Geometry: see drawing. Coordinates: mm, zero at the bounding-box minimum. Coordinates: 2 decimals unless noted, no trailing zeros. Write each loop counter-clockwise with the first axis right and the second up, starting at its lowest first coordinate (ties: lowest second). Pieces come first, ordered by that corner, then holes. Notation, with made-up numbers: (36, -4.75) - (42, -4.75) arc R25 ccw to (42, 32.25) - close; hole circle Ø7 at (-11, 29). An arc over 180 degrees is marked (long way). Use CSV: the item, a comma, the result in double quotes.
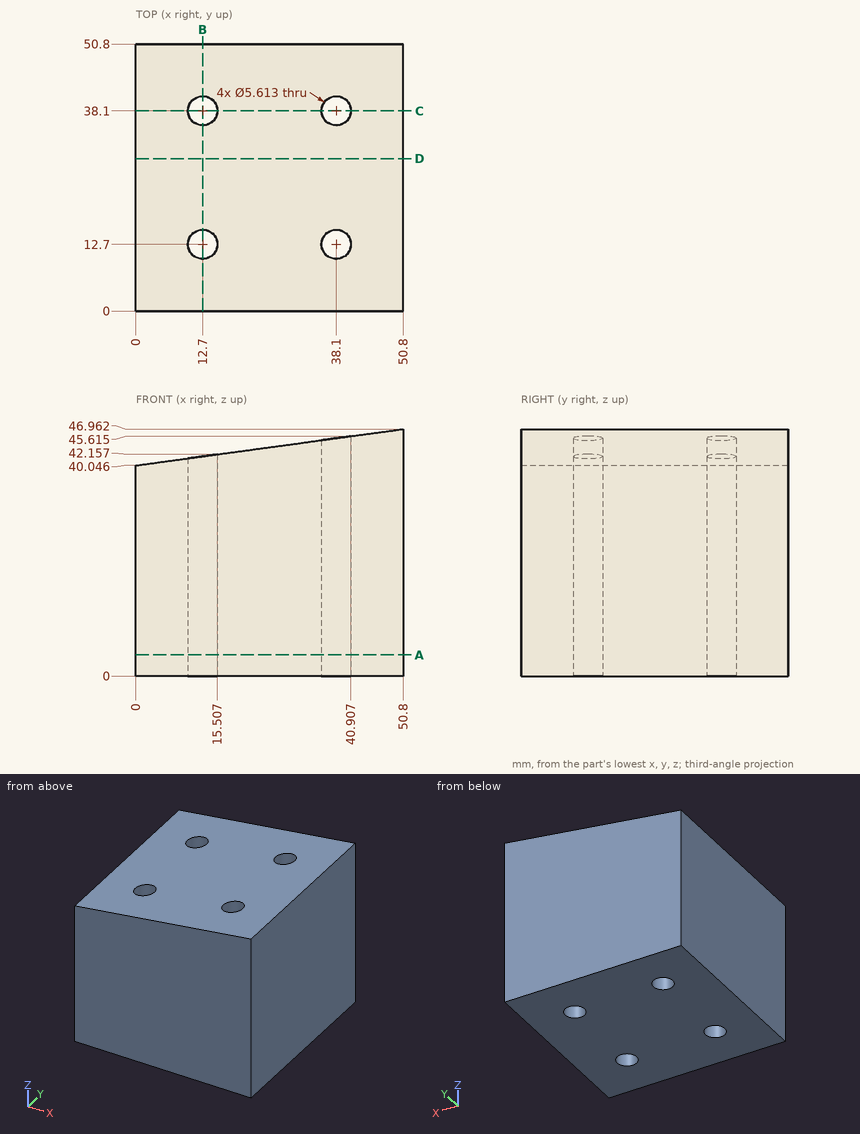
(1) Cut plane C-C on y = 38.1. State how many separate pieces and enclosed holes the cut face has, and give its area (3 significant figures).
Check values:
separate pieces,"3"
enclosed holes,"0"
area,"1,720 mm^2"
(2) Ray query, probe 1 along X at (y, z) = (12.7, 26); probe 2 along Y at (x, z) = (14, 38). Return the intervals inside material, ascending. Write a range as from..to.
Check values:
probe 1,"0..9.89, 15.51..35.29, 40.91..50.8"
probe 2,"0..10.21, 15.19..35.61, 40.59..50.8"
(3) Cut plane D-D on y = 29. Return loops of the section in (x, z), and give its area (3 significant figures).
Check values:
outline,"(0, 0) - (50.8, 0) - (50.8, 46.96) - (0, 40.05) - close"
area,"2,210 mm^2"
(4) Cut plane A-A on z = 4. Return loops of the section in (x, y), and give its area (3 significant figures).
Check values:
outline,"(0, 0) - (50.8, 0) - (50.8, 50.8) - (0, 50.8) - close; hole circle Ø5.61 at (12.7, 12.7); hole circle Ø5.61 at (12.7, 38.1); hole circle Ø5.61 at (38.1, 12.7); hole circle Ø5.61 at (38.1, 38.1)"
area,"2,480 mm^2"
(5) Pin query (flat end, axial travel): pin 1 Ø6.5 at (x, y) = (12.7, 38.1) entering from +Z; pin 2 Ø5 at (x, y) = (10, 36) entering from +Z (1 decimal); pin 3 Ø5 at (x, y) = (28.5, 16.5) entering from +Z. Return the tip coordinate at first contact, or that it passes through.
Check values:
pin 1,"z = 42.22"
pin 2,"z = 41.7"
pin 3,"z = 44.27"
(6) Cut plane B-B on x = 12.7. Return loops of the section in (y, z) (1 decimal).
Check values:
outline,"(0, 0) - (9.9, 0) - (9.9, 41.8) - (0, 41.8) - close; (15.5, 0) - (35.3, 0) - (35.3, 41.8) - (15.5, 41.8) - close; (40.9, 0) - (50.8, 0) - (50.8, 41.8) - (40.9, 41.8) - close"
